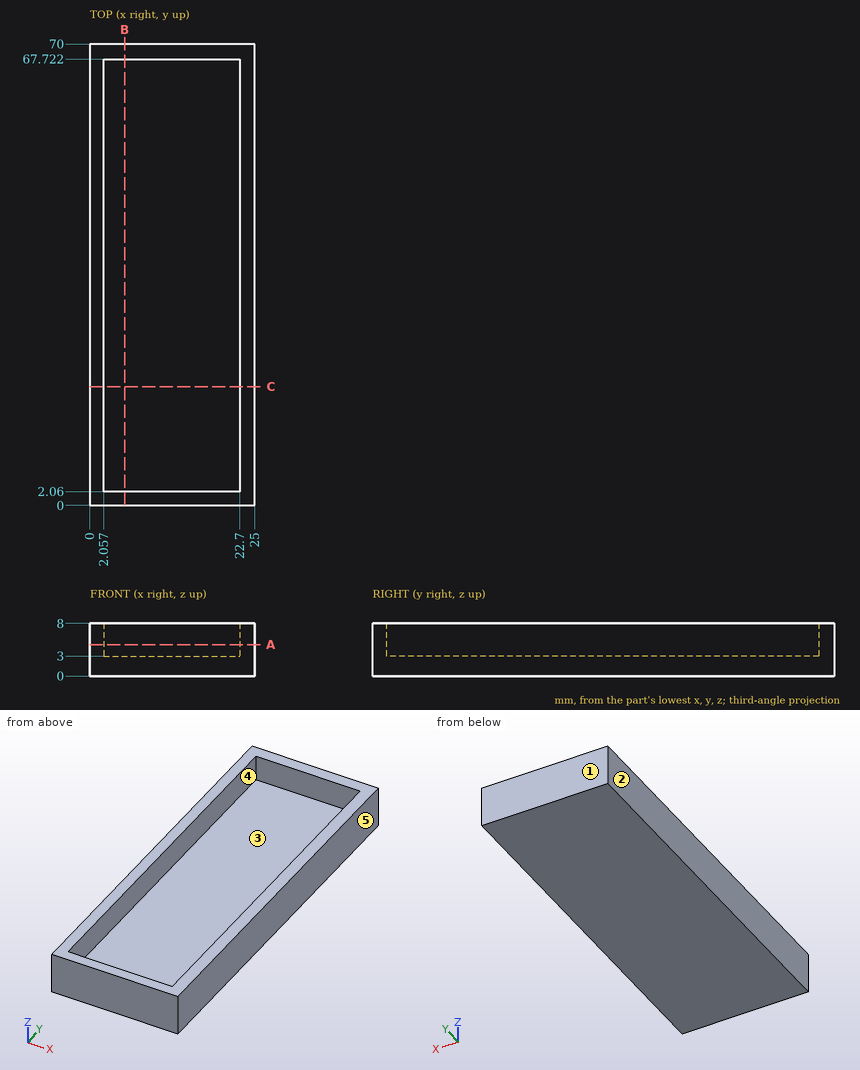
Drawing for the job (mm, zero at the part's lowest x, y, z). A direction names the side the tool comes from. Give positions to 0.01 mm unless a question says otherwise; leave off trailing zeros. Loops run counter-clockwise (first coordinate to the right, second up) from the corner with the lowest first, then second, coordinate; pieces in that order, holes last. Notation, with made-up numbers: M 77,53 L 124,53 A29 ccw 124,83 Z; hole C -12.75,-10 d6. An arc over 180 degrees is marked long. Use one line per item in the form item = value.
Item 1: Slice it at B-B (x = 5.25). List the corners of the cut face in (y, z), plus the area to 3 significant figures.
Determined:
outline = M 0,0 L 70,0 L 70,8 L 67.72,8 L 67.72,3 L 2.06,3 L 2.06,8 L 0,8 Z
area = 232 mm2
Item 2: Which spindle directions (+Z, -Z, +X, -X, +Y, -Y) get a long thin tool onto all of the face, cutting with end or side? Do the marked faces 4 and 5. Say none if no direction does.
Determined:
face_4 = +Z
face_5 = +Z, -Z, +X, +Y, -Y
Item 3: Two-plate mould, pull along X, no slides. Class the marked faces 1, 2 and 3: pulls with the +X half, pulls with the -X half, needs draft (parallel to the pull), parting line crosses it, or undercut.
Determined:
face_1 = needs draft
face_2 = pulls with the -X half
face_3 = undercut
Item 4: Slice it at A-A (z = 4.75). List the corners of the cut face in (x, y).
Determined:
outline = M 0,0 L 25,0 L 25,70 L 0,70 Z; hole M 2.06,2.06 L 22.7,2.06 L 22.7,67.72 L 2.06,67.72 Z
Item 5: Flat gauge pin, fed straight in: pin 1 (8 mm diameter, centred on x = 18, y = 47, fed in from +Z). Where does the tip first touch, or does it go through?
Determined:
pin_1 = 3
Item 6: Slice it at C-C (y = 18). List the corners of the cut face in (x, z).
Determined:
outline = M 0,0 L 25,0 L 25,8 L 22.7,8 L 22.7,3 L 2.06,3 L 2.06,8 L 0,8 Z
Item 7: Drill centre lines: probe 1 along X at (y, z) = (6, 6.75); probe 2 along Y at (x, z) = (6, 4); probe 3 along Z at (x, y) = (13.5, 9.5). Where is each one in solid material? Low to high. Write a range as from..to.
Determined:
probe_1 = 0..2.06, 22.7..25
probe_2 = 0..2.06, 67.72..70
probe_3 = 0..3
